Geometry: final body of the model. Coordinates: model frame, mm. A direction names the side the tool comes from. Give positions to 0.01 mm unless a question says otherwise; leave off trailing zeros. Order: outer loops, then holes, each group sorted by start corner. A loop starts at its lowest first (then second) coordinate and runs counter-clockwise, first axis right, second up. Notation, with made-up numbers: M 89.25,16 L 140.25,16 A27 cw 140.25,38 Z; hole C -7.5,69.5 d3. An arc over 180 degrees is marked long. Use CSV: the item, a comma, the result in double quotes.
```python
from build123d import *

# Parameters (mm, degrees)
SKETCH1_W           = 40.5
SKETCH1_H           = 34.5
BOSS_EXTRUDE1_DEPTH = 115
SKETCH2_R           = 1.5
SKETCH2_W           = 10
SKETCH2_H           = 2
BOSS_EXTRUDE2_DEPTH = 10
FILLET1_R           = 2


with BuildPart() as part:
    # Sketch1 → Boss-Extrude1 (new body)
    with BuildSketch(Plane(origin=(0, 0, 0), x_dir=(1, 0, 0), z_dir=(0, 1, 0))):
        Rectangle(SKETCH1_W, SKETCH1_H)
    extrude(amount=BOSS_EXTRUDE1_DEPTH)

    # Sketch2 → Boss-Extrude2 (add)
    with BuildSketch(Plane(origin=(0, 115, 0), x_dir=(1, 0, 0), z_dir=(0, 1, 0))):
        with Locations(Location((-15, 15.25, 0), (0, 0, 90))):
            Circle(SKETCH2_R)
        with Locations(Location((15, 15.25, 0), (0, 0, 90))):
            Circle(SKETCH2_R)
        with Locations((0, 15.25)):
            Rectangle(SKETCH2_W, SKETCH2_H)
    extrude(amount=BOSS_EXTRUDE2_DEPTH)

    # Fillet1
    fillet1_edges = [part.edges().sort_by_distance(p)[0] for p in [
        (-20.25, 115, 0),
        (20.25, 115, 0),
        (-20.25, 0, 0),
        (20.25, 0, 0),
    ]]
    fillet(fillet1_edges, radius=FILLET1_R)


solid = part.part
```
1. Reachability of faces 1 (the face through (-20.25, 57, 0)), 2 (the face through (0, 120, -14.25)), 3 (the face through (14.93, 119.93, -13.75)) from +Z, -Z, +X, -X, +Y, -Y: full face, straight path, thin tool, end or side. Return the list, or none.
Answer:
face 1,"+Z, -Z, -X, +Y, -Y"
face 2,"+Z, +Y"
face 3,"+Y"
2. Pull-direction query (X, two-part tool) for faces 4 (the face through (0, 57, -17.25)), 5 (the face through (0, 120, -16.25)), 6 (the face through (20.25, 57, 0)); classes: +X half, -X half, draft (parallel to the pull), parting line (faces both ways), or undercut.
Answer:
face 4,"draft"
face 5,"undercut"
face 6,"+X half"
3. Pin query (flat end, axial travel): pin 1 Ø1.5 at (x, z) = (-14, 7.5) entering from +Y; pin 2 Ø2 at (y, z) = (122, -15) entering from -X; pin 3 Ø2 at (y, z) = (121.5, -15.5) entering from +X. Return the tip coordinate at first contact, or that it passes through.
Answer:
pin 1,"y = 115"
pin 2,"x = -16.5"
pin 3,"x = 16.5"
4. Line query: line 1 (Y direction, x = -9.5, z = -2); line 2 (Z direction, x = -14, y = 119). Output: solid intervals per line, ascending.
Answer:
line 1,"0 to 115"
line 2,"-16.37 to -14.13"
5. Section B-B, the plane z = 8. Return the cut outline in (x, y).
Answer:
outline,"M -20.25,2 A2 ccw -18.25,0 L 18.25,0 A2 ccw 20.25,2 L 20.25,113 A2 ccw 18.25,115 L -18.25,115 A2 ccw -20.25,113 Z"
6. Section A-A, the plane x = -15. Return the cut outline in (y, z).
Answer:
outline,"M 0,-17.25 L 115,-17.25 L 115,-16.75 L 125,-16.75 L 125,-13.75 L 115,-13.75 L 115,17.25 L 0,17.25 Z"
